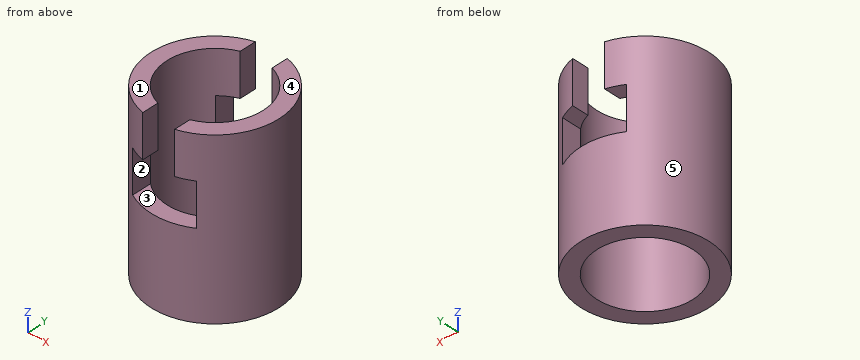
```python
from build123d import *

# Parameters (mm, degrees)
F0_R     = 30
F0_R_2   = 22.5
F1_DEPTH = 80
F3_DEPTH = 30


with BuildPart() as f1:
    # F0 (on Top) → F1 (new body)
    with BuildSketch(Plane.XY):
        Circle(F0_R)
        Circle(F0_R_2, mode=Mode.SUBTRACT)
    extrude(amount=F1_DEPTH)

    # F2 (on Front) → F3 (cut, symmetric)
    with BuildSketch(Plane.XZ):
        Polygon((-7.5, 60), (-15, 60), (-15, 40), (15, 40), (15, 60), (7.5, 60), (7.5, 80), (-7.5, 80), align=None)
    extrude(amount=F3_DEPTH, both=True, mode=Mode.SUBTRACT)


solid = f1.part
```
Build history of the part. All positions in model axes, mm. Face numbers are marked on the shaded views. A direction names the side the tool comes from. Coordinates: 2 decimals unless noted, no trailing zeros. Order: outer loops, then holes, each group sorted by start corner. A loop starts at its lowest first (then second) coordinate and runs counter-clockwise, first axis right, second up.
Item 1: Drill centre lines: L1, parallel to Y at x = 0, z = 38; L2, parallel to Z at x = -14, y = 25; L3, parallel to Y at x = 9.5, z = 68. Where is each one in solid material? Low to high.
Filled in:
L1: y = -30 to -22.5, 22.5 to 30
L2: z = 0 to 40, 60 to 80
L3: y = -28.46 to -20.4, 20.4 to 28.46
Item 2: Tool access for the marked faces 1 and 2: list every direction of +Z, -Z, +X, -X, +Y, -Y with a clear straight run to the whole face (end or side of a thin tool).
Filled in:
face 1: +Z, +X, -X, +Y, -Y
face 2: +Y, -Y
Item 3: Saw through at B-B on z = 59. List the corners of the cut face in (x, y).
Filled in:
outline: (-15, -25.98) - (-15, -16.77) arc R22.5 cw to (-15, 16.77) - (-15, 25.98) arc R30 ccw to start; (15, -25.98) arc R30 ccw to (15, 25.98) - (15, 16.77) arc R22.5 cw to (15, -16.77) - close
Item 4: Drop flat-ended pins along their axis: pin 1 Ø3 at (x, z) = (1.5, 38) entering from +Y; pin 2 Ø3 at (y, z) = (7.5, 46) entering from -X; pin 3 Ø2.5 at (y, z) = (-26.5, 70.5) entering from +X. Give the stop position or say it passes through.
Filled in:
pin 1: stops at y = 30
pin 2: stops at x = -29.39
pin 3: stops at x = 16.2
Item 5: Saw through at A-A on x = 0. List the corners of the cut face in (y, z).
Filled in:
outline: (-30, 0) - (-22.5, 0) - (-22.5, 40) - (-30, 40) - close; (22.5, 0) - (30, 0) - (30, 40) - (22.5, 40) - close
Item 6: Mould opens along X. For the marked faces 3, 4 and 5 say: released by +X, released by -X, zero draft, split by the parting line, or undercut.
Filled in:
face 3: undercut
face 4: zero draft
face 5: split by the parting line
Item 7: Saw through at C-C on x = 11. List the corners of the cut face in (y, z).
Filled in:
outline: (-27.91, 0) - (-19.63, 0) - (-19.63, 40) - (-27.91, 40) - close; (-27.91, 60) - (-19.63, 60) - (-19.63, 80) - (-27.91, 80) - close; (19.63, 0) - (27.91, 0) - (27.91, 40) - (19.63, 40) - close; (19.63, 60) - (27.91, 60) - (27.91, 80) - (19.63, 80) - close
Item 8: Saw through at D-D on y = 25. List the corners of the cut face in (x, z), then the cut area to 3 significant figures.
Filled in:
outline: (-16.58, 0) - (16.58, 0) - (16.58, 80) - (7.5, 80) - (7.5, 60) - (15, 60) - (15, 40) - (-15, 40) - (-15, 60) - (-7.5, 60) - (-7.5, 80) - (-16.58, 80) - close
area: 1,750 mm2
